from build123d import *

# Parameters (mm, degrees)
SKETCH1_R           = 11.25
SKETCH1_R_2         = 2
BOSS_EXTRUDE1_DEPTH = 8
SKETCH2_R           = 2.125
CUT_EXTRUDE1_DEPTH  = 18.808003819
SKETCH3_R           = 4.15
CUT_EXTRUDE2_DEPTH  = 2
CUT_EXTRUDE3_START  = -1.5
SKETCH4_R           = 11.25
SKETCH4_R_2         = 9.9
CUT_EXTRUDE3_DEPTH  = 1.5


with BuildPart() as part:
    # Sketch1 → Boss-Extrude1 (new body)
    with BuildSketch(Plane(origin=(0, 0, 0), x_dir=(1, 0, 0), z_dir=(0, 1, 0))):
        with Locations(Location((0, 0, 0), (0, 0, 270))):
            Circle(SKETCH1_R)
        with Locations(Location((0, 0, 0), (0, 0, 270))):
            Circle(SKETCH1_R_2, mode=Mode.SUBTRACT)
    extrude(amount=BOSS_EXTRUDE1_DEPTH)

    # Sketch2 → Cut-Extrude1 (cut, through all)
    with BuildSketch(Plane.XZ):
        with Locations(Location((-7.6, 0, 0), (0, 0, 270))):
            Circle(SKETCH2_R)
        with Locations(Location((3.8, 6.581793069, 0), (0, 0, 270))):
            Circle(SKETCH2_R)
        with Locations(Location((3.8, -6.581793069, 0), (0, 0, 270))):
            Circle(SKETCH2_R)
    extrude(amount=-CUT_EXTRUDE1_DEPTH, mode=Mode.SUBTRACT)

    # Sketch3 → Cut-Extrude2 (cut)
    with BuildSketch(Plane.XZ):
        with Locations((-7.6, 0)):
            Circle(SKETCH3_R)
        with Locations((3.8, 6.581793069)):
            Circle(SKETCH3_R)
        with Locations((3.8, -6.581793069)):
            Circle(SKETCH3_R)
    extrude(amount=-CUT_EXTRUDE2_DEPTH, mode=Mode.SUBTRACT)

    # Sketch4 → Cut-Extrude3 (cut)
    with BuildSketch(Plane(origin=(0, 8, 0), x_dir=(1, 0, 0), z_dir=(0, 1, 0)).offset(CUT_EXTRUDE3_START)):
        with Locations(Location((0, 0, 0), (0, 0, 72.260290628))):
            Circle(SKETCH4_R)
        with Locations(Location((0, 0, 0), (0, 0, 270))):
            Circle(SKETCH4_R_2, mode=Mode.SUBTRACT)
    extrude(amount=CUT_EXTRUDE3_DEPTH, mode=Mode.SUBTRACT)


solid = part.part
Model file for the job. Use its own axes, mm. A direction names the side the tool comes from. Give positions to 0.01 mm unless a question says otherwise; leave off trailing zeros. Order: outer loops, then holes, each group sorted by start corner. A loop starts at its lowest first (then second) coordinate and runs counter-clockwise, first axis right, second up. Notation, with made-up numbers: M 21,-38.5 L 29,-38.5 A23 cw 29,-14.5 Z; hole C -22,-9.5 d4. An arc over 180 degrees is marked long. Write item = value, one per line.
Q1. Cut at A-A, the plane z = 0. List the corners of the cut face in (x, y) (3 decimals).
Derived:
outline = M -11.25,2 L -9.725,2 L -9.725,8 L -9.9,8 L -9.9,6.5 L -11.25,6.5 Z; M -5.475,2 L -3.45,2 L -3.45,0 L -2,0 L -2,8 L -5.475,8 Z; M 2,0 L 11.25,0 L 11.25,6.5 L 9.9,6.5 L 9.9,8 L 2,8 Z
Q2. Cut at D-D, the plane x = 0. List the corners of the cut face in (y, z), then the cut area to 3 significant figures.
Derived:
outline = M 0,-11.25 L 6.5,-11.25 L 6.5,-9.9 L 8,-9.9 L 8,-2 L 0,-2 L 0,-4.91 L 2,-4.91 L 2,-8.25 L 0,-8.25 Z; M 0,2 L 8,2 L 8,9.9 L 6.5,9.9 L 6.5,11.25 L 0,11.25 L 0,8.25 L 2,8.25 L 2,4.91 L 0,4.91 Z
area = 131 mm2
Q3. Cut at B-B, the plane x = 3.8. List the corners of the cut face in (y, z), then the cut area to 3 significant figures.
Derived:
outline = M 0,-2.43 L 2,-2.43 L 2,-4.46 L 8,-4.46 L 8,4.46 L 2,4.46 L 2,2.43 L 0,2.43 Z; M 2,-10.59 L 6.5,-10.59 L 6.5,-9.14 L 8,-9.14 L 8,-8.71 L 2,-8.71 Z; M 2,8.71 L 8,8.71 L 8,9.14 L 6.5,9.14 L 6.5,10.59 L 2,10.59 Z
area = 81.5 mm2
Q4. Flat gauge pins, fed straight in: pin 1 (1.5 mm diameter, centred on x = 4.5, y = 3, fed in from -Z); pin 2 (3 mm diameter, centred on y = 3, z = 3, fed in from +X); pin 3 (1.5 mm diameter, centred on x = -7, y = 2, fed in from -Z). Where does each tip first touch, or does it go through?
Derived:
pin_1 = -10.61
pin_2 = 11.15
pin_3 = -9.35
Q5. Drill centre lines: line 1 (Z direction, x = 3, y = 1); line 2 (Y direction, x = 8.5, z = 5.25); line 3 (Z direction, x = 3.8, y = 0.4). Where is each one in solid material? Low to high. Write a range as [from, to].
Derived:
line_1 = [-10.84, -10.65], [-2.51, 2.51], [10.65, 10.84]
line_2 = [0, 6.5]
line_3 = [-2.43, 2.43]
Q6. Tool access for faces 4 (the cylindrical face through (2.974, 7.24, 9.443)), 5 (the flat face through (-2.2, 0, -0.2)), 6 (the cylindrical face through (1.599, 0.986, 3.063)): list every direction of +Z, -Z, +X, -X, +Y, -Y with a clear straight run to the whole face (end or side of a thin tool).
Derived:
face_4 = +Y
face_5 = +Z, -Z, +X, -X, -Y
face_6 = -Y
Q7. Two-plate mould, pull along X, no slides. Class faces 1 (the flat face through (10, 6.5, 2)), 2 (the cylindrical face through (3.38, 3.2, 10.73)), 3 (the cylindrical face through (1.85, 0.99, -2.92)): pulls with the +X half, pulls with the -X half, needs draft (parallel to the pull), parting line crosses it, or undercut.
Derived:
face_1 = needs draft
face_2 = parting line crosses it
face_3 = undercut
Q8. Cut at C-C, the plane y = 7. List the corners of the cut face in (x, z) (3 decimals), then the cut area to 3 significant figures.
Derived:
outline = C 0,0 d19.8; hole C -7.6,0 d4.25; hole C 0,0 d4; hole C 3.8,-6.582 d4.25; hole C 3.8,6.582 d4.25
area = 253 mm2
